The drawing under review shows one solid part. Ordinate dimensions are in mm from its lowest x, y, z. A direction names the side the tool comes from. Coordinates: 2 decimals unless noted, no trailing zeros. Order: outer loops, then holes, each group sorted by start corner. A loop starts at its lowest first (then second) coordinate and runs counter-clockwise, first axis right, second up. Notation, with made-up numbers: M -0.5,46 L 43.5,46 A22 cw 43.5,84 Z; hole C -9.75,-38.5 d6. An arc over 180 degrees is marked long. Answer as a JSON object with one key per item and string values.
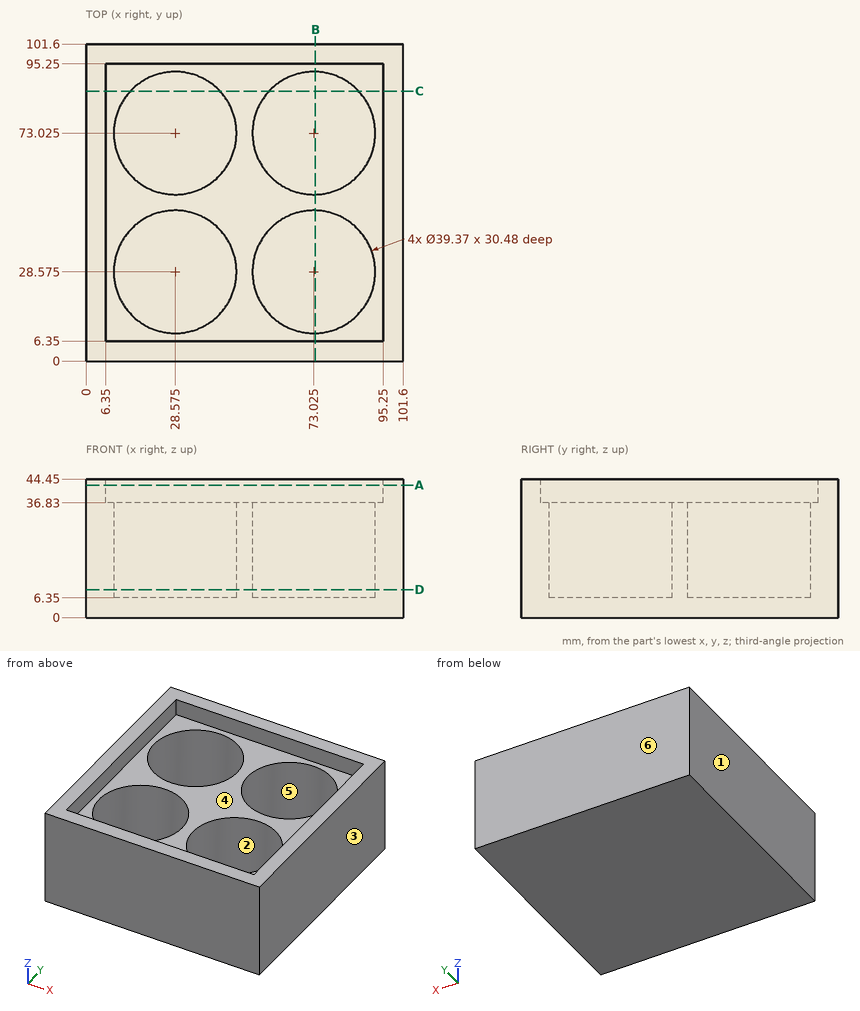
1) Tool access review of the marked faces 1 and 2: name each direction out of +Z, -Z, +X, -X, +Y, -Y from which nothing blocks a thin tool from reaching the whole face with its end or side.
Taken from the geometry:
{"face 1": "+Z, -Z, -X, +Y, -Y", "face 2": "+Z"}
2) Insertion check: pin 1 Ø6 at (x, y) = (62, 37.5) entering from -Z; pin 2 Ø10 at (x, y) = (88, 49.5) entering from +Z; pin 3 Ø23.5 at (x, y) = (73.025, 73.025) entering from +Z. Each pin has a flat end and moves straight along its axis. Give the tip position at first contact, or say it passes through.
Taken from the geometry:
{"pin 1": "stops at z = 0", "pin 2": "stops at z = 36.83", "pin 3": "stops at z = 6.35"}
3) Add section B-B (x = 73.5). State the section outline as (y, z) points, and give its area (3 significant figures).
Taken from the geometry:
{"outline": "M 0,0 L 101.6,0 L 101.6,44.45 L 95.25,44.45 L 95.25,36.83 L 92.7,36.83 L 92.7,6.35 L 53.35,6.35 L 53.35,36.83 L 48.25,36.83 L 48.25,6.35 L 8.9,6.35 L 8.9,36.83 L 6.35,36.83 L 6.35,44.45 L 0,44.45 Z", "area": "1,440 mm2"}
4) Add section C-C (y = 86.5). State the section outline as (x, z) points, and give its area (3 significant figures).
Taken from the geometry:
{"outline": "M 0,0 L 101.6,0 L 101.6,44.45 L 95.25,44.45 L 95.25,36.83 L 87.38,36.83 L 87.38,6.35 L 58.67,6.35 L 58.67,36.83 L 42.93,36.83 L 42.93,6.35 L 14.22,6.35 L 14.22,36.83 L 6.35,36.83 L 6.35,44.45 L 0,44.45 Z", "area": "2,090 mm2"}
5) Mouldability with a two-part tool opening along Y and no side actions: class the marked faces 3, 4, 5 and 6 as released by +Y, released by -Y, zero draft, split by the parting line, or undercut.
Taken from the geometry:
{"face 3": "zero draft", "face 4": "undercut", "face 5": "undercut", "face 6": "released by +Y"}
6) Add section A-A (z = 42.5). State the section outline as (x, y) points, and give its area (3 significant figures).
Taken from the geometry:
{"outline": "M 0,0 L 101.6,0 L 101.6,101.6 L 0,101.6 Z; hole M 6.35,6.35 L 95.25,6.35 L 95.25,95.25 L 6.35,95.25 Z", "area": "2,420 mm2"}
7) Add section D-D (z = 9). State the section outline as (x, y) points (3 decimals), and give its area (3 significant figures).
Taken from the geometry:
{"outline": "M 0,0 L 101.6,0 L 101.6,101.6 L 0,101.6 Z; hole C 28.575,28.575 d39.37; hole C 28.575,73.025 d39.37; hole C 73.025,28.575 d39.37; hole C 73.025,73.025 d39.37", "area": "5,450 mm2"}
8) To check wall thickness, follow L1, parallel to X at y = 14.5, z = 41; L2, parallel to X at y = 16.5, z = 8. State the ranges of each line that lie inside material, in increasing order.
Taken from the geometry:
{"L1": "x = 0 to 6.35, 95.25 to 101.6", "L2": "x = 0 to 13.03, 44.12 to 57.48, 88.57 to 101.6"}
